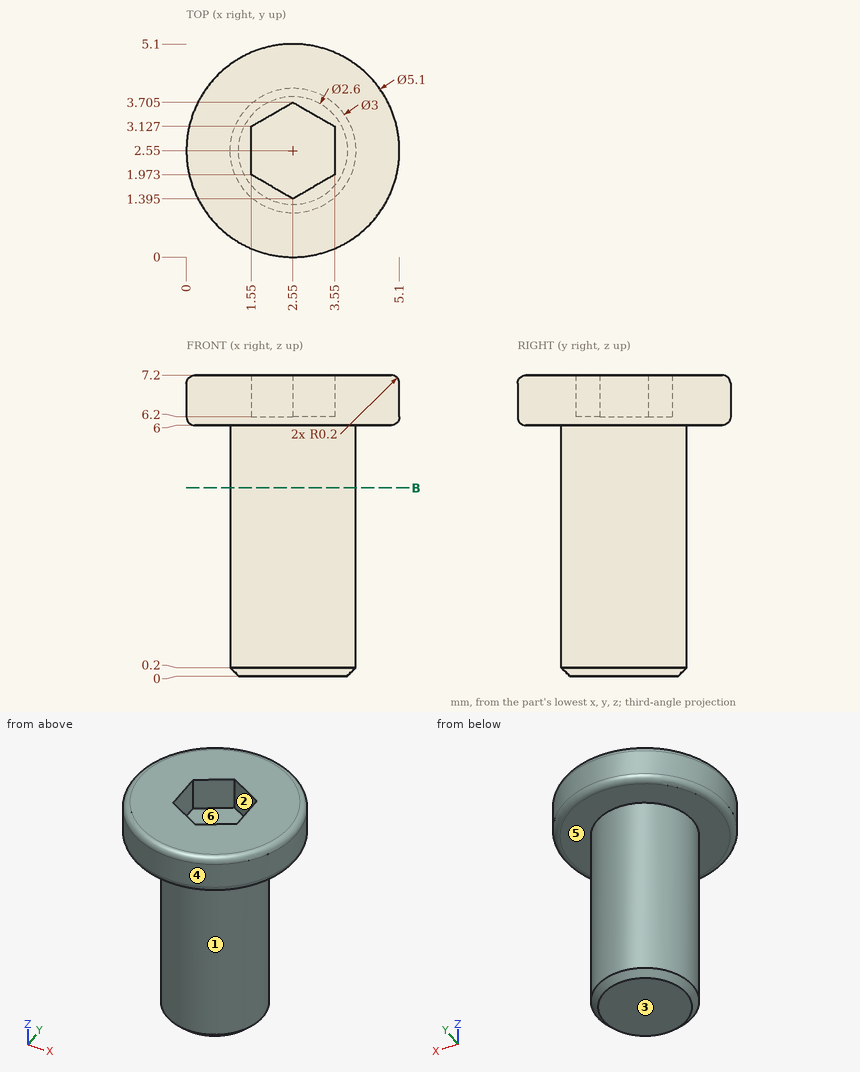
Here's the drawing with two shaded views (mm, measured from the low corner). I have some questions. A direction names the side the tool comes from. Give positions to 0.01 mm unless a question says otherwise; leave off trailing zeros. Write each loop counter-clockwise with the first axis right and the second up, starting at its lowest first coordinate (ties: lowest second). Pieces come first, ordered by that corner, then holes. Notation, with made-up numbers: (49.5, 26) -> (89.5, 26) arc R38 ccw to (89.5, 64) -> close; hole circle Ø4 at (63, 47.25). An arc over 180 degrees is marked (long way). Answer as a JSON object with one key per item and string values. Group by question number.
Item 1: For the marked faces 1, 2 and 3, which set-ups out of +Z, -Z, +X, -X, +Y, -Y let a thin tool reach every point of the face, with its end or its side?
Item 2: Please list where these lines run through material, in increasing order: line 1 (Z direction, x = 1.65, y = 3.05); line 2 (Z direction, x = 4.25, y = 3.35); line 3 (Y direction, x = 2.5, z = 1). Write a range as [from, to].
Item 3: I'm going to push a flat-ended pin straight in: P1, Ø1, axis at x = 1.5, z = 2.5, coming from the +Y side (1 decimal). Where does the tip first touch, or does it pass through?
Item 4: We'd pull the mould along Y, two halves only. Please class the marked faces 4, 5 and 6: +Y half, -Y half, draft (parallel to the pull), parting line (faces both ways), or undercut.
Item 5: Suppose I cut it at B-B (z = 4.5). Please give me the cut outline in (x, y).
Findings:
{
 "1": {"face 1": "-Z", "face 2": "+Z", "face 3": "-Z, +X, -X, +Y, -Y"},
 "2": {"line 1": "z = [0, 6.2]", "line 2": "z = [6, 7.2]", "line 3": "y = [1.05, 4.05]"},
 "3": {"P1": "stops at y = 3.9"},
 "4": {"face 4": "parting line", "face 5": "draft", "face 6": "undercut"},
 "5": {"outline": "circle Ø3 at (2.55, 2.55)"}
}
